The model under review builds one solid part; all positions refer to its coordinate system, in mm. Face numbers are marked on the shaded views. Coordinates: 2 decimals unless noted, no trailing zeros. Loops run counter-clockwise (first coordinate to the right, second up) from the corner with the lowest first, then second, coordinate; pieces in that order, holes last. Notation, with made-up numbers: M 18.25,83 L 31.25,83 A19 ccw 31.25,102 Z; hole C 8,84.25 d8. An arc over 180 degrees is marked long. One line per item, written item: value.
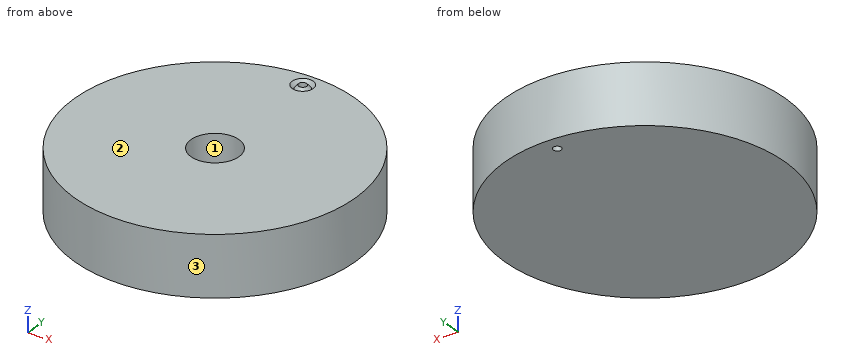
```python
from build123d import *

# Parameters (mm, degrees)
F0_R     = 44.45
F1_DEPTH = 19.05
F2_R     = 7.62
F3_DEPTH = 12.7
F4_R     = 1.27
F5_DEPTH = 19.051
F6_R     = 3.3274
F6_R_2   = 1.27
F7_DEPTH = 2.1082
F7_TAPER = 41


with BuildPart() as f1:
    # F0 (on Top) → F1 (new body)
    with BuildSketch(Plane.XY):
        Circle(F0_R)
    extrude(amount=F1_DEPTH)

    # F2 (on face) → F3 (cut)
    with BuildSketch(Plane.XY.offset(19.05)):
        Circle(F2_R)
    extrude(amount=-F3_DEPTH, mode=Mode.SUBTRACT)

    # F4 (on face) → F5 (cut, through all)
    with BuildSketch(Plane.XY.offset(19.05)):
        with Locations((0, 39.6875)):
            Circle(F4_R)
    extrude(amount=-F5_DEPTH, mode=Mode.SUBTRACT)

    # F6 (on face) → F7 (cut)
    with BuildSketch(Plane.XY.offset(19.05)):
        with Locations((0, 39.6875)):
            Circle(F6_R)
        with Locations((0, 39.6875)):
            Circle(F6_R_2, mode=Mode.SUBTRACT)
    extrude(amount=-F7_DEPTH, taper=F7_TAPER, mode=Mode.SUBTRACT)


solid = f1.part
```
(1) Add section A-A on x = 0. State the section outline as (y, z) points, then the cut area to 3 significant figures.
Checks:
outline: M -44.45,0 L 38.42,0 L 38.42,19.05 L 37.39,17.87 L 36.36,19.05 L 7.62,19.05 L 7.62,6.35 L -7.62,6.35 L -7.62,19.05 L -44.45,19.05 Z; M 40.96,0 L 44.45,0 L 44.45,19.05 L 43.01,19.05 L 41.99,17.87 L 40.96,19.05 Z
area: 1,450 mm^2
(2) Insertion check: pin 1 Ø4.5 at (x, y) = (-1.5, 1) entering from +Z; pin 2 Ø6 at (y, z) = (-14, 4) entering from +X; pin 3 Ø1.5 at (y, z) = (-8.5, 14.5) entering from -X; pin 4 Ø2 at (x, y) = (0, 39.69) entering from -Z. Each pin has a flat end and moves straight along its axis. Give the tip position at first contact, or say it passes through.
Checks:
pin 1: z = 6.35
pin 2: x = 43.07
pin 3: x = -43.77
pin 4: through
(3) Add section D-D on x = 18.5. State the section outline as (y, z) points.
Checks:
outline: M -40.42,0 L 40.42,0 L 40.42,19.05 L -40.42,19.05 Z
(4) Draft analysis for pull direction X (two halves, no side actions). For the marked faces 1, 2 and 3, state which applies: pulls with the +X half, pulls with the -X half, needs draft (parallel to the pull), parting line crosses it, or undercut.
Checks:
face 1: undercut
face 2: needs draft
face 3: parting line crosses it
(5) To check wall thickness, follow L1, parallel to Y at x = 0, z = 8.75; L2, parallel to Y at x = 0, z = 5; L3, parallel to Z at x = -1, y = -2.5. State the ranges of each line that lie inside material, in increasing order. Write a range as [from, to].
Checks:
L1: [-44.45, -7.62], [7.62, 38.42], [40.96, 44.45]
L2: [-44.45, 38.42], [40.96, 44.45]
L3: [0, 6.35]
(6) Add section B-B on y = 0. State the section outline as (x, z) points, then the cut area to 3 significant figures.
Checks:
outline: M -44.45,0 L 44.45,0 L 44.45,19.05 L 7.62,19.05 L 7.62,6.35 L -7.62,6.35 L -7.62,19.05 L -44.45,19.05 Z
area: 1,500 mm^2
(7) Add section C-C on z = 9.5. State the section outline as (x, y) points, then the cut area to 3 significant figures.
Checks:
outline: C 0,0 d88.9; hole C 0,0 d15.24; hole C 0,39.69 d2.54
area: 6,020 mm^2
